The listing builds one solid part. Answer for the finished solid, in the listing's coordinates (mm). A direction names the side the tool comes from. Give positions to 0.01 mm unless a question says otherwise; leave off trailing zeros. Order: outer loops, then holes, each group sorted by start corner. A loop starts at its lowest first (then second) coordinate and runs counter-clockwise, first axis right, second up. Notation, with made-up numbers: (85.25, 13.5) - (99.25, 13.5) arc R29 ccw to (99.25, 44.5) - close; hole circle Ø9 at (31, -2.75). An arc over 180 degrees is marked (long way). Write each question's results on one line, items separated by ' | '. Start each with the question number.
1. Flat-ended cylindrical pins translate along their axes: pin 1 (4 mm diameter, centred on x = 7, y = 21.5, fed in from -Z); pin 2 (1.7 mm diameter, centred on x = 48, y = 48, fed in from +Z); pin 3 (6.5 mm diameter, centred on x = -47, y = 61.5, fed in from -Z); pin 4 (14 mm diameter, centred on x = -6.5, y = 55.5, fed in from -Z). Find the tip coordinate at first contact, or state that the pin passes through.
2. Find the intervals of material crossed by L1, parallel to X at y = 48, z = 0; L2, parallel to X at y = 41, z = -32; L3, parallel to Z at x = -63, y = 61, in increasing order.
3. Section A-A (y = 56) is taken. Give the vertices of the cut face in (x, z).
4. Which of the six approach directions +Z, -Z, +X, -X, +Y, -Y give full straight-line access (tool end or side, diameter ignored) to faces 1 (the face through (-29.506, 50.689, 57.308)), 2 (the face through (29.443, 0.386, 57.779)), 3 (the face through (-29.7, 99.62, 57.64))?
5. Section B-B (z = 0) is taken. State how many separate pieces and enclosed holes the cut face has, and give its area (3 significant figures).
from build123d import *

# Parameters (mm, degrees)
HOLDER_SECTION_PROFILE_R    = 73.787
HOLDER_SECTION_BODY_DEPTH   = 100
PAYLOAD_HOLE_PROFILE_W      = 101
PAYLOAD_HOLE_PROFILE_H      = 101
PAYLOAD_HOLE_CUT_DEPTH      = 145.530421497
ACCESS_HOLE_CUT_DEPTH       = 145.530421497
FILLET1_R                   = 12.7
THREADED_ROD_HOLE_PROFILE_R = 3.3782
THREADED_ROD_HOLE_CUT_DEPTH = 145.530421497
CHAMFER1_SIZE               = 0.762


with BuildPart() as part:
    # Holder Section Profile → Holder Section Body (new body)
    with BuildSketch(Plane(origin=(0, 0, 0), x_dir=(1, 0, 0), z_dir=(0, 1, 0))):
        with Locations(Location((0, 0, 0), (0, 0, 270))):
            Circle(HOLDER_SECTION_PROFILE_R)
    extrude(amount=HOLDER_SECTION_BODY_DEPTH)

    # Payload Hole Profile → Payload Hole Cut (cut, through all)
    with BuildSketch(Plane(origin=(0, 100, 0), x_dir=(1, 0, 0), z_dir=(0, 1, 0))):
        Rectangle(PAYLOAD_HOLE_PROFILE_W, PAYLOAD_HOLE_PROFILE_H)
    extrude(amount=-PAYLOAD_HOLE_CUT_DEPTH, mode=Mode.SUBTRACT)

    # Access Hole Profile → Access Hole Cut (cut, through all)
    with BuildSketch(Plane(origin=(0, 100, 0), x_dir=(1, 0, 0), z_dir=(0, 1, 0))):
        Polygon((-17.4625, -64.2619994), (17.4625, -64.2619994), (41.298982175, -50.5), (-41.298982175, -50.5), align=None)
    access_hole_cut = extrude(amount=-ACCESS_HOLE_CUT_DEPTH, mode=Mode.SUBTRACT)

    # Access Hole Mirror: Access Hole Cut across plane
    add(access_hole_cut.mirror(Plane(origin=(0, 0, 0), x_dir=(1, 0, 0), z_dir=(0, 0, -1))), mode=Mode.SUBTRACT)

    # Fillet1
    fillet1_edges = [part.edges().sort_by_distance(p)[0] for p in [
        (-17.4625, 50, 64.2619994),
        (-41.298982175, 50, 50.5),
        (41.298982175, 50, 50.5),
        (17.4625, 50, 64.2619994),
        (-41.298982175, 50, -50.5),
        (-17.4625, 50, -64.2619994),
        (17.4625, 50, -64.2619994),
        (41.298982175, 50, -50.5),
    ]]
    fillet(fillet1_edges, radius=FILLET1_R)

    # Threaded Rod Hole Profile → Threaded Rod Hole Cut (cut, through all)
    with BuildSketch(Plane(origin=(0, 100, 0), x_dir=(1, 0, 0), z_dir=(0, 1, 0))):
        with Locations(Location((-63.5, 0, 0), (0, 0, 270))):
            Circle(THREADED_ROD_HOLE_PROFILE_R)
        with Locations(Location((63.5, 0, 0), (0, 0, 270))):
            Circle(THREADED_ROD_HOLE_PROFILE_R)
    extrude(amount=-THREADED_ROD_HOLE_CUT_DEPTH, mode=Mode.SUBTRACT)

    # Chamfer1
    chamfer1_edges = [part.edges().sort_by_distance(p)[0] for p in [
        (50.5, 0, 0),
        (-47.600968459, 0, 50.5),
        (-50.5, 0, 0),
        (47.600968459, 0, -50.5),
        (50.5, 100, 0),
        (-63.5, 0, -3.3782),
        (-63.5, 100, -3.3782),
        (63.5, 0, -3.3782),
        (47.600968459, 100, -50.5),
        (63.5, 100, -3.3782),
        (-50.5, 100, 0),
        (-47.600968459, 100, 50.5),
        (0, 0, -73.787),
        (0, 100, -73.787),
        (29.380741087, 100, 57.3809997),
        (29.380741087, 0, 57.3809997),
        (0, 100, 64.2619994),
        (0, 0, 64.2619994),
        (47.600968459, 0, 50.5),
        (47.600968459, 100, 50.5),
        (-47.600968459, 100, -50.5),
        (-29.380741087, 100, -57.3809997),
        (0, 100, -64.2619994),
        (29.380741087, 100, -57.3809997),
        (-29.380741087, 100, 57.3809997),
        (-41.414935046, 100, -50.932742006),
        (41.414935046, 100, -50.932742006),
        (-41.414935046, 100, 50.932742006),
        (41.414935046, 100, 50.932742006),
        (-29.380741087, 0, -57.3809997),
        (-47.600968459, 0, -50.5),
        (-29.380741087, 0, 57.3809997),
        (29.380741087, 0, -57.3809997),
        (0, 0, -64.2619994),
        (-41.414935046, 0, -50.932742006),
        (41.414935046, 0, -50.932742006),
        (-41.414935046, 0, 50.932742006),
        (41.414935046, 0, 50.932742006),
        (17.346547129, 100, 63.829257394),
        (17.346547129, 0, 63.829257394),
        (-17.346547129, 100, 63.829257394),
        (-17.346547129, 0, 63.829257394),
        (17.346547129, 100, -63.829257394),
        (17.346547129, 0, -63.829257394),
        (-17.346547129, 100, -63.829257394),
        (-17.346547129, 0, -63.829257394),
    ]]
    chamfer(chamfer1_edges, length=CHAMFER1_SIZE)


solid = part.part
Reported:
1) pin 1: z = -73.62 | pin 2: z = 56.76 | pin 3: z = -59.42 | pin 4: z = -73.79
2) L1: -73.79 to -66.88, -60.12 to -50.5, 50.5 to 60.12, 66.88 to 73.79 | L2: -66.49 to -50.5, 50.5 to 66.49 | L3: -38.41 to -3.34, 3.34 to 38.41
3) outline: circle Ø147.57 at (0, 0); hole circle Ø6.76 at (-63.5, 0); hole (-50.5, -50.5) - (-44.7, -50.5) arc R12.7 cw to (-38.35, -52.2) - (-20.41, -62.56) arc R12.7 ccw to (-14.06, -64.26) - (14.06, -64.26) arc R12.7 ccw to (20.41, -62.56) - (38.35, -52.2) arc R12.7 cw to (44.7, -50.5) - (50.5, -50.5) - (50.5, 50.5) - (44.7, 50.5) arc R12.7 cw to (38.35, 52.2) - (20.41, 62.56) arc R12.7 ccw to (14.06, 64.26) - (-14.06, 64.26) arc R12.7 ccw to (-20.41, 62.56) - (-38.35, 52.2) arc R12.7 cw to (-44.7, 50.5) - (-50.5, 50.5) - close; hole circle Ø6.76 at (63.5, 0)
4) face 1: +Y, -Y | face 2: -Y | face 3: +Y
5) separate pieces: 4 | enclosed holes: 0 | area: 3,300 mm²
